Build history of the part. All positions in model axes, mm. Face numbers are marked on the shaded views. A direction names the side the tool comes from. Coordinates: 2 decimals unless noted, no trailing zeros. Order: outer loops, then holes, each group sorted by start corner. A loop starts at its lowest first (then second) coordinate and runs counter-clockwise, first axis right, second up. Notation, with made-up numbers: M 77.25,-28.5 L 85.25,-28.5 A18 cw 85.25,-11.5 Z; hole C 75.25,10 d2. An arc over 180 degrees is marked long. Use a Markdown table: item, result. Add a question column.
from build123d import *

# Parameters (mm, degrees)
SKETCH1_W                = 52
SKETCH1_H                = 75
BOSS_EXTRUDE1_DEPTH      = 3
BOSS_EXTRUDE2_DEPTH      = 38
BOSS_EXTRUDE2_DEPTH_BACK = 40
SKETCH2_W                = 2.5
SKETCH2_H                = 75
SKETCH5_W                = 75
SKETCH5_H                = 3
BOSS_EXTRUDE5_DEPTH      = 47
CUT_EXTRUDE1_DEPTH       = 92.643201899
CUT_EXTRUDE1_DEPTH_BACK  = 92.643201899
SKETCH6_W                = 47
SKETCH6_H                = 3
CHAMFER1_SIZE            = 5


with BuildPart() as part:
    # Sketch1 → Boss-Extrude1 (new body)
    with BuildSketch(Plane(origin=(0, 0, 0), x_dir=(1, 0, 0), z_dir=(0, 1, 0))):
        with Locations((-7.052631579, -5.043859649)):
            Rectangle(SKETCH1_W, SKETCH1_H)
    extrude(amount=BOSS_EXTRUDE1_DEPTH)

    # Sketch2 → Boss-Extrude2 (add, two sides: drawn at the far end of the back side and taken through both)
    with BuildSketch(Plane(origin=(0, 3, 0), x_dir=(1, 0, 0), z_dir=(0, 1, 0)).offset(-BOSS_EXTRUDE2_DEPTH_BACK)):
        with Locations((-31.802631579, -5.043859649)):
            Rectangle(SKETCH2_W, SKETCH2_H)
        with Locations((17.697368421, -5.043859649)):
            Rectangle(SKETCH2_W, SKETCH2_H)
    extrude(amount=BOSS_EXTRUDE2_DEPTH + BOSS_EXTRUDE2_DEPTH_BACK)

    # Sketch5 → Boss-Extrude5 (add)
    with BuildSketch(Plane(origin=(-30.552631579, 0, 0), x_dir=(0, 0, -1), z_dir=(1, 0, 0))):
        with Locations((-5.043859649, 22.5)):
            Rectangle(SKETCH5_W, SKETCH5_H)
    extrude(amount=BOSS_EXTRUDE5_DEPTH)

    # Sketch6 → Cut-Extrude1 (cut, two sides: drawn at the far end of the back side and taken through both)
    with BuildSketch(Plane.XY.offset(42.543859649).offset(-CUT_EXTRUDE1_DEPTH_BACK)):
        with Locations((-7.052631579, 1.5)):
            Rectangle(SKETCH6_W, SKETCH6_H)
    extrude(amount=CUT_EXTRUDE1_DEPTH + CUT_EXTRUDE1_DEPTH_BACK, mode=Mode.SUBTRACT)

    # Chamfer1
    chamfer1_edges = [part.edges().sort_by_distance(p)[0] for p in [
        (-31.802631579, 41, 42.543859649),
        (-31.802631579, 41, -32.456140351),
        (17.697368421, 41, -32.456140351),
        (17.697368421, 41, 42.543859649),
    ]]
    chamfer(chamfer1_edges, length=CHAMFER1_SIZE)


solid = part.part
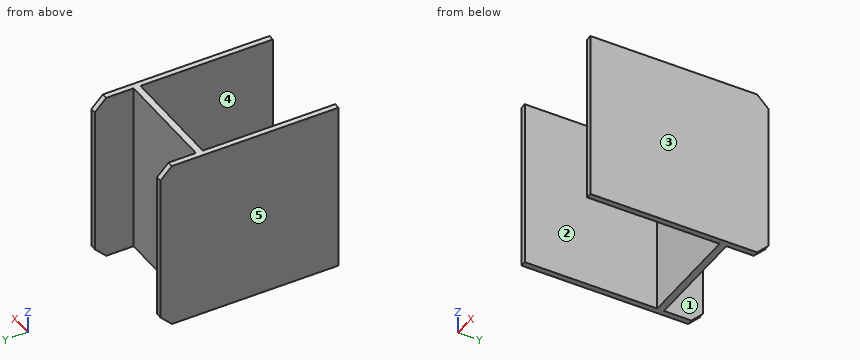
(1) Drill centre lines: line 1 along X through (y, z) = (-8.5, -16); line 2 along Y through (x, z) = (-13, -1.5); line 3 along Y through (x, z) = (16.5, 38). Where is each one in solid material? Low to high. Write a range as from..to.
(2) Which spindle directions (+Z, -Z, +X, -X, +Y, -Y) get a long thin tool onto all of the face, cutting with end or side? Do the marked faces 1 and 2. Say none if no direction does.
(3) Drop flat-ended pins along their axis: P1, Ø14, axis at x = 1.5, z = -12.5, coming from the +Y side; P2, Ø2, axis at x = -3, z = -15.5, coming from the -Y side. Give the stop position or say it passes through.
(4) Mould opens along X. For the marked faces 3, 4 and 5 say: released by +X, released by -X, zero draft, split by the parting line, or undercut.
(5) Slice it at B-B on z = -23.5. Give the cut face in (x, y).
(6) Slice it at C-C on x = -23. Give the cut face in (y, z), and give its area (3 significant figures).
(7) Slice it at A-A on y = -26. Give the cut face in (x, z), and give its area (3 significant figures).
Solutions:
| question | item | result |
|---|---|---|
| 1 | line 1 | -33.05..-30.55, 16.45..18.95 |
| 1 | line 2 | 21..24 |
| 1 | line 3 | -37..40.54 |
| 2 | face 1 | +Z, -Z, +Y |
| 2 | face 2 | +Z, -Z, -Y |
| 3 | P1 | y = 24 |
| 3 | P2 | y = 21 |
| 4 | face 3 | released by +X |
| 4 | face 4 | undercut |
| 4 | face 5 | released by -X |
| 5 | outline | M -33.05,-37 L -30.55,-37 L -30.55,21 L 16.45,21 L 16.45,-37 L 18.95,-37 L 18.95,41 L 16.45,41 L 16.45,24 L -30.55,24 L -30.55,41 L -33.05,41 Z |
| 6 | outline | M 21,-32.46 L 24,-32.46 L 24,42.54 L 21,42.54 Z |
| 6 | area | 225 mm² |
| 7 | outline | M -33.05,-32.46 L -30.55,-32.46 L -30.55,42.54 L -33.05,42.54 Z; M 16.45,-32.46 L 18.95,-32.46 L 18.95,42.54 L 16.45,42.54 Z |
| 7 | area | 375 mm² |
